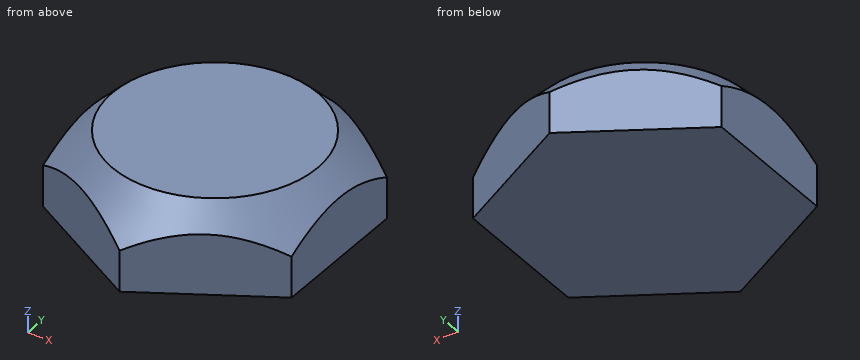
```python
from build123d import *

# Parameters (mm, degrees)
SKETCH_R          = 3.5
PAD_DEPTH         = 2
CHAMFER_SIZE      = 1
SKETCH001_R       = 4.5
POCKET_DEPTH      = 2.001
POCKET_DEPTH_BACK = 0.001


with BuildPart() as part:
    # Sketch → Pad (new body)
    with BuildSketch(Plane.XY):
        Circle(SKETCH_R)
    extrude(amount=PAD_DEPTH)

    # Chamfer
    chamfer_edges = [part.edges().sort_by_distance(p)[0] for p in [
        (-3.5, 0, 2),
    ]]
    chamfer(chamfer_edges, length=CHAMFER_SIZE)

    # Sketch001 (on Face3 of Pad) → Pocket (cut, two sides)
    with BuildSketch(Plane.XY.offset(2)) as pocket_sk:
        Circle(SKETCH001_R)
        Polygon((3.031089, 1.75), (0, 3.5), (-3.031089, 1.75), (-3.031089, -1.75), (0, -3.5), (3.031089, -1.75), align=None, mode=Mode.SUBTRACT)
    extrude(amount=-POCKET_DEPTH, mode=Mode.SUBTRACT)
    extrude(pocket_sk.sketch, amount=POCKET_DEPTH_BACK, mode=Mode.SUBTRACT)


solid = part.part
```
For this review, take the finished solid that the model builds, in its own axes (mm). Coordinates: 2 decimals unless noted, no trailing zeros. Loops run counter-clockwise (first coordinate to the right, second up) from the corner with the lowest first, then second, coordinate; pieces in that order, holes last.
1. Insertion check: P1, Ø1, axis at y = 2.5, z = 1.5, coming from the -X side. The pin has a flat end and moves straight along its axis. Give the tip position at first contact, or say it passes through.
2. Add section A-A, the plane z = 1.55. Give the boundary of the cut face in (x, y).
3. For line 1 (Z direction, x = 0, y = 2.75); line 2 (Y direction, x = -0.25, z = 0.6); line 3 (Z direction, x = 1, y = 2.75), list the stretches that pass through material, from the lowest coordinate up.
4. Add section B-B, the plane z = 0.75. Give the boundary of the cut face in (x, y), then the cut area to 3 significant figures.
Result:
1. P1: stops at x = -2.5
2. outline: circle Ø5.9 at (0, 0)
3. line 1: z = 0 to 1.75
3. line 2: y = -3.36 to 3.36
3. line 3: z = 0 to 1.57
4. outline: (-3.03, -1.75) - (0, -3.5) - (3.03, -1.75) - (3.03, 1.75) - (0, 3.5) - (-3.03, 1.75) - close
4. area: 31.8 mm2
